Verification items for this drawing (mm, ordinates from the low corner). A direction names the side the tool comes from. Round coordinates to 2 decimals unless told otherwise and drop trailing zeros. Order: outer loops, then holes, each group sorted by start corner. A loop starts at its lowest first (then second) coordinate and runs counter-clockwise, first axis right, second up. Notation, with made-up numbers: (19, -11) -> (67, -11) arc R19 ccw to (67, 13) -> close; hole circle Ø4 at (13.25, -8). An arc over 180 degrees is marked (long way). Use a Markdown table: item, result. Add a question column.
Item 1: Mould release check, pull along Y, two halves, no side actions. Record for the marked faces 3 and 4: pulls with the +Y half, pulls with the -Y half, needs draft (parallel to the pull), parting line crosses it, or undercut.
Item 2: Set-up check for the marked faces 1 and 2: record each of +Z, -Z, +X, -X, +Y, -Y from which the full face is reachable in a straight line by a thin tool's end or side.
Item 3: Sectioned sample at A-A, the plane x = 17.88. Record the cut outline in (y, z) (3 decimals), and give its area (3 significant figures).
Item 4: Sectioned sample at C-C, the plane x = 33. Record the cut outline in (y, z).
Item 5: Material ranges on probe 1 along Z at (x, y) = (28, 12.5); probe 2 along X at (y, z) = (17, 7.5); probe 3 along Z at (x, y) = (20.5, 17.5), recorded low to high. Write a range as [from, to].
Item 6: Gauge pin test, flat ends, axial feed: pin 1 Ø9 at (x, y) = (17, 25) entering from +Z; pin 2 Ø12 at (x, y) = (32.5, 8.5) entering from -Z; pin 3 Ø2 at (y, z) = (21.5, 6.5) entering from -X. Record the tip position at first contact, or that the pin passes through.
Item 7: Sectioned sample at B-B, the plane z = 26.5. Record the cut outline in (x, y), and give its area (3 significant figures).
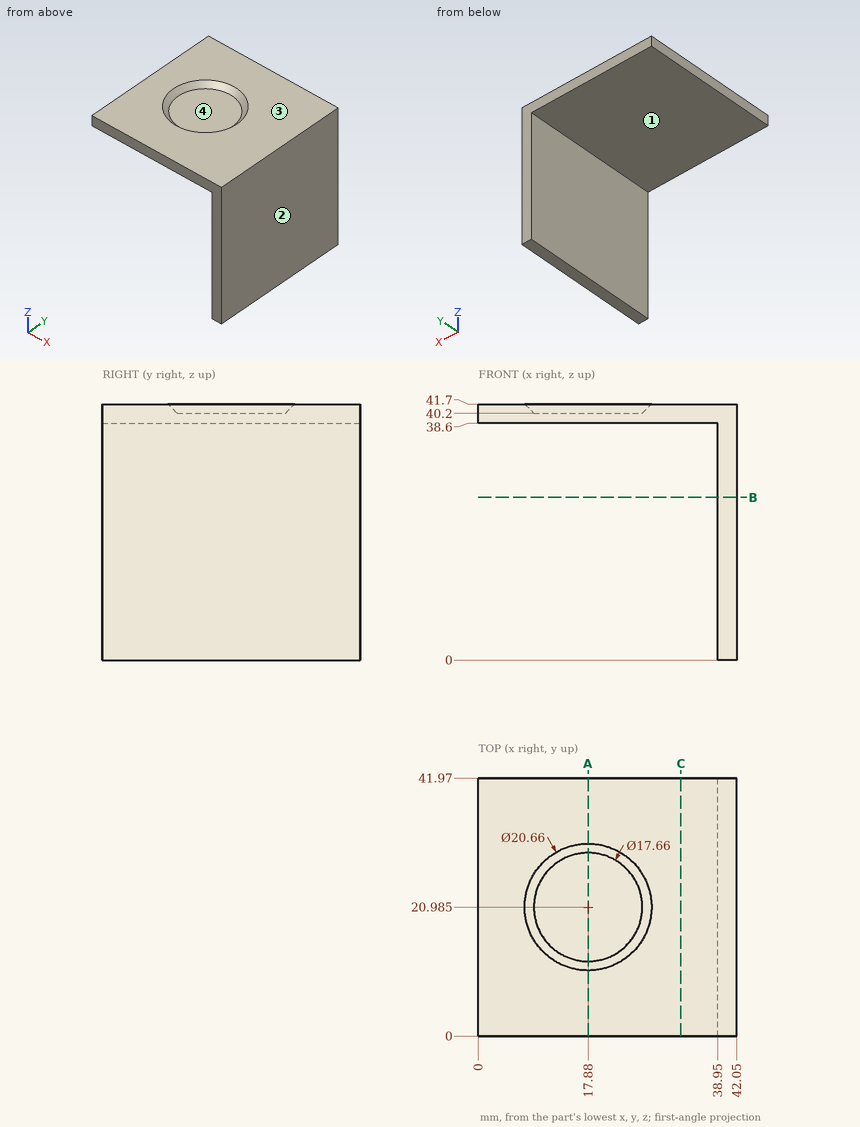
Found:
| question | item | result |
|---|---|---|
| 1 | face 3 | needs draft |
| 1 | face 4 | undercut |
| 2 | face 1 | -Z, -X, +Y, -Y |
| 2 | face 2 | +Z, -Z, +X, +Y, -Y |
| 3 | outline | (0, 38.6) -> (41.97, 38.6) -> (41.97, 41.7) -> (31.315, 41.7) -> (29.815, 40.2) -> (12.155, 40.2) -> (10.655, 41.7) -> (0, 41.7) -> close |
| 3 | area | 101 mm2 |
| 4 | outline | (0, 38.6) -> (41.97, 38.6) -> (41.97, 41.7) -> (0, 41.7) -> close |
| 5 | probe 1 | z = [38.6, 41.7] |
| 5 | probe 2 | x = [38.95, 42.05] |
| 5 | probe 3 | z = [38.6, 40.2] |
| 6 | pin 1 | stops at z = 40.2 |
| 6 | pin 2 | stops at z = 38.6 |
| 6 | pin 3 | stops at x = 38.95 |
| 7 | outline | (38.95, 0) -> (42.05, 0) -> (42.05, 41.97) -> (38.95, 41.97) -> close |
| 7 | area | 130 mm2 |
